Model file for the job. Use its own axes, mm. Give positions to 0.01 mm unless a question says otherwise; leave off trailing zeros. Write each loop counter-clockwise with the first axis right and the second up, starting at its lowest first coordinate (ties: lowest second). Pieces come first, ordered by that corner, then holes.
```python
from build123d import *

# Parameters (mm, degrees)
F2_R     = 116.9838211005
F3_DEPTH = 25
F4_W     = 276.3622701168
F4_H     = 252.8828978539
F5_DEPTH = 25


# Not quite as in the source:
# - the program builds the solid bodies; features that only make, move or delete a surface that nothing else refers to are left out


with BuildPart() as f3:
    # F2 (on Right) → F3 (new body)
    with BuildSketch(Plane.YZ):
        Circle(F2_R)
    extrude(amount=F3_DEPTH)

    # F4 (on Front) → F5 (join)
    with BuildSketch(Plane.XZ):
        with Locations((138.1811350584, 148.9392518997)):
            Rectangle(F4_W, F4_H)
    extrude(amount=F5_DEPTH)


solid = f3.part
```
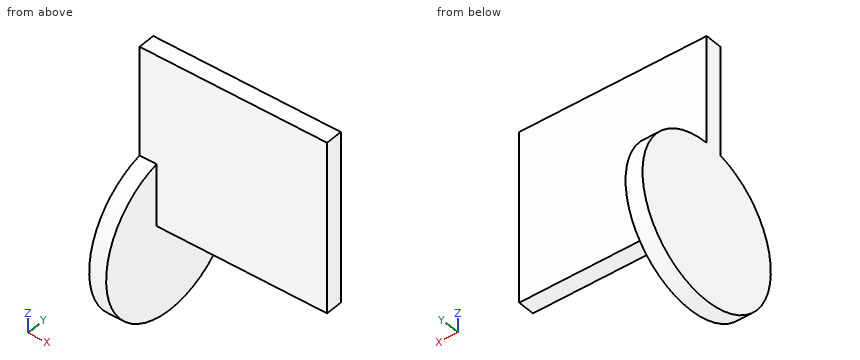
1. Slice it at A-A, the plane z = 64. Write the cut outline in (x, y).
Calculated:
outline: (0, -97.92) - (25, -97.92) - (25, -25) - (276.36, -25) - (276.36, 0) - (25, 0) - (25, 97.92) - (0, 97.92) - close
2. Slice it at C-C, the plane y = -40. Write the cut outline in (x, z).
Calculated:
outline: (0, -109.93) - (25, -109.93) - (25, 109.93) - (0, 109.93) - close
3. Slice it at B-B, the plane x = 210. Write the cut outline in (y, z).
Calculated:
outline: (-25, 22.5) - (0, 22.5) - (0, 275.38) - (-25, 275.38) - close
4. Probe probe 1 along Y at (x, z) = (70, 154); probe 2 along X at (y, z) = (87, -58); probe 3 along Z at (x, y) = (20, -60.5). List the from-to ranges inside material, lowest first.
Calculated:
probe 1: y = -25 to 0
probe 2: x = 0 to 25
probe 3: z = -100.12 to 100.12
5. Pin check, flat tips, straight feed: P1, Ø20, axis at x = 207.5, y = -15, coming from the -Z side; P2, Ø8, axis at x = 175.5, z = 159.5, coming from the +Y side; P3, Ø1.5, axis at x = 215, z = 21.5, coming from the +Y side; P4, Ø1, axis at x = 115, z = 40, coming from the -Y side. Stop position of each tip, or through.
Calculated:
P1: stops at z = 22.5
P2: stops at y = 0
P3: passes through
P4: stops at y = -25
